Autodesk Inventor part; units mm, degrees
ref_plane "YZ Plane" through (0, 0, 0) normal (1, 0, 0) x (0, 1, 0)
ref_plane "XZ Plane" through (0, 0, 0) normal (0, 1, 0) x (-1, 0, 0)
ref_plane "XY Plane" through (0, 0, 0) normal (0, 0, 1) x (1, 0, 0)
sketch "스케치1" plane through (0, 0, 0) normal (0, 1, 0) x (-1, 0, 0)
  line L0 (103, 0) -> (93, 0)
  line L1 (0, 0) -> (0, -91)
  line L2 (0, -91) -> (103, -91)
  line L3 (103, -91) -> (103, 0)
  line L4 (93, -91) -> (93, -96)
  line L5 (93, -96) -> (16, -96)
  line L6 (16, -96) -> (16, -91)
  line L7 (93, 0) -> (0, 0)
  line L8 (103, -5) -> (0, -5)
  line L9 (5, 0) -> (5, -91)
  line L10 (0, -86) -> (103, -86)
  line L11 (95, 0) -> (95, -91)
  point P0 (93, -93.5)
  point P1 (16, -93.5)
  point P2 (51.5, -86)
  point P3 (95, -5)
  point P4 (95, -86)
  point P5 (5, -86)
  point P6 (5, -5)
  dimension "d0" = 103
  dimension "d1" = 91
  dimension "d2" = 5
  dimension "d3" = 10
  dimension "d4" = 16
  dimension "d5" = 8
  dimension "d6" = 5
  dimension "d7" = 5
  dimension "d8" = 5
extrude "돌출1" add sketch "스케치1" along normal blind 21 contours L3 L8 L11 L0 | L11 L8 L9 L7 L0 | L3 L10 L11 L8 | L3 L2 L11 L10 | L9 L8 L1 L7 | L9 L10 L1 L8 | L11 L2 L9 L10 | L9 L2 L1 L10 | L4 L5 L6 L2
extrude "돌출2" add sketch "스케치1" along normal blind 6 contours L11 L10 L9 L8
sketch "스케치2" plane through (0, 21, 0) normal (0, 1, 0) x (1, 0, 0)
  line L0 (-16, 96) -> (-93, 96)
  line L1 (-21, 96) -> (-21, 86)
  line L2 (-95, 86) -> (-5, 86)
  line L3 (-88, 96) -> (-88, 76.7304)
  line L4 (-93, 96) -> (-93, 91)
  line L5 (-16, 91) -> (-16, 96)
  point P0 (0, 0)
  point P1 (-93, 93.5)
  point P2 (-88, 86)
  dimension "d13" = 5
  dimension "d14" = 5
extrude "돌출3" cut sketch "스케치2" against normal blind 16
properties part number "imu"
Build history of the part. All positions in model axes, mm. A direction names the side the tool comes from. Round coordinates to 2 decimals unless told otherwise and drop trailing zeros. Order: outer loops, then holes, each group sorted by start corner. A loop starts at its lowest first (then second) coordinate and runs counter-clockwise, first axis right, second up. Notation, with made-up numbers: (-18, 14.25) -> (38, 14.25) arc R23 ccw to (38, 47.25) -> close; hole circle Ø10 at (56, 41). An arc over 180 degrees is marked (long way). Answer in a Markdown table with one row per item.
1) Band-saw the part on B-B on z = -59. Give the cut face in (x, y), and give its area (3 significant figures).
Values:
| item | result |
|---|---|
| outline | (-103, 0) -> (0, 0) -> (0, 21) -> (-5, 21) -> (-5, 6) -> (-95, 6) -> (-95, 21) -> (-103, 21) -> close |
| area | 813 mm2 |
2) Band-saw the part on C-C on y = 13.5. Give the cut face in (x, z), and give its area (3 significant figures).
Values:
| item | result |
|---|---|
| outline | (-103, -91) -> (-93, -91) -> (-93, -96) -> (-88, -96) -> (-88, -86) -> (-95, -86) -> (-95, -5) -> (-5, -5) -> (-5, -86) -> (-21, -86) -> (-21, -96) -> (-16, -96) -> (-16, -91) -> (0, -91) -> (0, 0) -> (-103, 0) -> close |
| area | 1,800 mm2 |
3) Mould opens along Z. For faces 1 (the flat face through (-55, 3, -96)), 2 (the flat face through (-13, 13, -86)), 3 (the flat face through (-21, 13, -91)) say: released by +Z, released by -Z, zero draft, split by the parting line, or undercut.
Values:
| item | result |
|---|---|
| face 1 | released by -Z |
| face 2 | undercut |
| face 3 | zero draft |
4) Pin check, flat tips, straight feed: P1, Ø2, axis at x = -92.5, z = -25.5, coming from the +Y side; P2, Ø2.5, axis at y = 5.5, z = -93.5, coming from the -X side; P3, Ø2, axis at x = -54, y = 12.5, coming from the -Z side. Stop position of each tip, or through.
Values:
| item | result |
|---|---|
| P1 | y = 6 |
| P2 | x = -93 |
| P3 | z = -5 |
5) Which spindle directions (+Z, -Z, +X, -X, +Y, -Y) get a long thin tool onto all of the face, cutting with end or side? Do faces 4 (the flat face through (0, 10, -45)), 5 (the flat face through (-8, 10, -91)), 6 (the flat face through (-93, 10, -93)), 7 (the flat face through (-88, 13, -91)), 8 (the flat face through (-95, 13, -45)). Say none if no direction does.
Values:
| item | result |
|---|---|
| face 4 | +Z, -Z, +X, +Y, -Y |
| face 5 | -Z, +X, +Y, -Y |
| face 6 | -Z, -X, +Y, -Y |
| face 7 | -Z, +Y |
| face 8 | +Y |
6) Band-saw the part on A-A on x = -55. Give the cut face in (y, z).
Values:
| item | result |
|---|---|
| outline | (0, -96) -> (5, -96) -> (5, -86) -> (6, -86) -> (6, -5) -> (21, -5) -> (21, 0) -> (0, 0) -> close |
7) Wall check: L1, parallel to X at y = 18, z = -13; L2, parallel to Z at x = -8.5, y = 11; L3, parallel to Y at x = -74.5, z = -89. Give the ranges that are in metal, low to high.
Values:
| item | result |
|---|---|
| L1 | -103 to -95, -5 to 0 |
| L2 | -91 to -86, -5 to 0 |
| L3 | 0 to 5 |
